Source: CAD feature listing. Evaluate the final solid. Frame: model axes, mm. A direction names the side the tool comes from. Give positions to 0.01 mm unless a question says otherwise; leave off trailing zeros. Loops run counter-clockwise (first coordinate to the right, second up) from the corner with the lowest first, then second, coordinate; pieces in that order, holes last. Notation, with made-up numbers: (47, -27.5) -> (56, -27.5) arc R18 ccw to (56, -3.5) -> close; hole circle Ø6 at (-22.5, 62). An arc over 180 degrees is marked (long way). Put each result on its own line as item: value.
```python
from build123d import *

# Parameters (mm, degrees)
SKETCH_1_W          = 74
SKETCH_1_H          = 42
SKETCH_1_R          = 1.275
EXTRUDE_1_DEPTH     = 2
SKETCH_2_R          = 1.525
CUT_EXTRUDE_1_DEPTH = 2
FILLET_1_R          = 2
SKETCH_3_W          = 30
SKETCH_3_H          = 22
EXTRUDE_2_DEPTH     = 2
SKETCH_4_R          = 2.025
CUT_EXTRUDE_2_DEPTH = 10
FILLET_2_R          = 2
CUT_EXTRUDE_3_DEPTH = 10
SKETCH_6_W          = 16
SKETCH_6_H          = 9
CUT_EXTRUDE_4_DEPTH = 10
FILLET_3_R          = 2


with BuildPart() as part:
    # 草图1 → 凸台-拉伸1 (new body)
    with BuildSketch(Plane.XY):
        Rectangle(SKETCH_1_W, SKETCH_1_H)
        with Locations((18, 18)):
            Circle(SKETCH_1_R, mode=Mode.SUBTRACT)
        with Locations((-18, 18)):
            Circle(SKETCH_1_R, mode=Mode.SUBTRACT)
        with Locations((-18, -18)):
            Circle(SKETCH_1_R, mode=Mode.SUBTRACT)
        with Locations((18, -18)):
            Circle(SKETCH_1_R, mode=Mode.SUBTRACT)
    extrude(amount=EXTRUDE_1_DEPTH)

    # 草图2 → 切除-拉伸1 (cut)
    with BuildSketch(Plane.XY.offset(2)):
        with Locations((34, 18)):
            Circle(SKETCH_2_R)
        with Locations((-34, 18)):
            Circle(SKETCH_2_R)
        with Locations((-34, -18)):
            Circle(SKETCH_2_R)
        with Locations((34, -18)):
            Circle(SKETCH_2_R)
    extrude(amount=-CUT_EXTRUDE_1_DEPTH, mode=Mode.SUBTRACT)

    # 圆角1
    fillet_1_edges = [part.edges().sort_by_distance(p)[0] for p in [
        (37, -21, 1),
        (-37, -21, 1),
        (-37, 21, 1),
        (37, 21, 1),
    ]]
    fillet(fillet_1_edges, radius=FILLET_1_R)

    # 草图3 → 凸台-拉伸2 (add)
    with BuildSketch(Plane.XY.offset(2)):
        with Locations((0, -21)):
            Rectangle(SKETCH_3_W, SKETCH_3_H)
    extrude(amount=-EXTRUDE_2_DEPTH)

    # 草图4 → 切除-拉伸2 (cut)
    with BuildSketch(Plane.XY.offset(2)):
        with Locations((12, -28)):
            Circle(SKETCH_4_R)
        with Locations((-12, -28)):
            Circle(SKETCH_4_R)
    extrude(amount=-CUT_EXTRUDE_2_DEPTH, mode=Mode.SUBTRACT)

    # 圆角2
    fillet_2_edges = [part.edges().sort_by_distance(p)[0] for p in [
        (15, -21, 1),
        (-15, -21, 1),
        (-15, -32, 1),
        (15, -32, 1),
    ]]
    fillet(fillet_2_edges, radius=FILLET_2_R)

    # 草图5 → 切除-拉伸3 (cut)
    with BuildSketch(Plane(origin=(0, 0, 0), x_dir=(-1, 0, 0), z_dir=(0, 0, -1))):
        Polygon((0, -2.18303115), (-27.010214515, -14), (27.010214515, -14), align=None)
        Polygon((-32, 11.81696885), (-32, -11.81696885), (-4.989785485, 0), align=None)
        Polygon((-27.010214515, 14), (0, 2.18303115), (27.010214515, 14), align=None)
        Polygon((32, 11.81696885), (4.989785485, 0), (32, -11.81696885), align=None)
    extrude(amount=-CUT_EXTRUDE_3_DEPTH, mode=Mode.SUBTRACT)

    # 草图6 → 切除-拉伸4 (cut)
    with BuildSketch(Plane(origin=(0, 0, 0), x_dir=(-1, 0, 0), z_dir=(0, 0, -1))):
        with Locations((0, -22.5)):
            Rectangle(SKETCH_6_W, SKETCH_6_H)
    extrude(amount=-CUT_EXTRUDE_4_DEPTH, mode=Mode.SUBTRACT)

    # 圆角3
    fillet_3_edges = [part.edges().sort_by_distance(p)[0] for p in [
        (0, 2.18303115, 1),
        (27.010214515, 14, 1),
        (-27.010214515, 14, 1),
        (32, -11.81696885, 1),
        (32, 11.81696885, 1),
        (4.989785485, 0, 1),
        (-4.989785485, 0, 1),
        (-32, 11.81696885, 1),
        (-32, -11.81696885, 1),
        (27.010214515, -14, 1),
        (0, -2.18303115, 1),
        (-27.010214515, -14, 1),
        (-8, -18, 1),
        (-8, -27, 1),
        (8, -27, 1),
        (8, -18, 1),
    ]]
    fillet(fillet_3_edges, radius=FILLET_3_R)


solid = part.part
```
(1) Draft query along Y for faces 3 (the flat face through (9.404, -6.297, 0.986)), 4 (the flat face through (-26, -21, 1)). Return one class per face: released by +Y, released by -Y, zero draft, split by the parting line, or undercut.
Calculated:
face 3: undercut
face 4: released by -Y
(2) Section B-B on x = -34. Return loops of the section in (y, z) (3 decimals), then the cut area to 3 significant figures.
Calculated:
outline: (-21, 0) -> (-19.525, 0) -> (-19.525, 2) -> (-21, 2) -> close; (-16.475, 0) -> (16.475, 0) -> (16.475, 2) -> (-16.475, 2) -> close; (19.525, 0) -> (21, 0) -> (21, 2) -> (19.525, 2) -> close
area: 71.8 mm²
(3) Section A-A on y = -28. Return loops of the section in (x, z) (3 decimals).
Calculated:
outline: (-15, 0) -> (-14.025, 0) -> (-14.025, 2) -> (-15, 2) -> close; (-9.975, 0) -> (9.975, 0) -> (9.975, 2) -> (-9.975, 2) -> close; (14.025, 0) -> (15, 0) -> (15, 2) -> (14.025, 2) -> close
(4) Reachability of faces 1 (the cylindrical face through (-31.07, -10.45, 1.01)), 2 (the cylindrical face through (36.4, -20.43, 1.01)) from +Z, -Z, +X, -X, +Y, -Y: full face, straight path, thin tool, end or side. Return the list, or none.
Calculated:
face 1: +Z, -Z
face 2: +Z, -Z, +X, -Y
(5) First-contact query: P1, Ø12, axis at x = -12, y = -16, coming from the -Z side; P2, Ø2, axis at x = -18, y = -18, coming from the +Z side; P3, Ø0.6, axis at x = -28.5, z = 1, coming from the -Y side; P4, Ø1, axis at y = -25, z = 1.5, coming from the +X side. Flat tips, straight axial feed; report the tip coordinate or a pass-through.
Calculated:
P1: stops at z = 0
P2: passes through
P3: stops at y = -21
P4: stops at x = 15
(6) Line query: probe 1 along Y at (x, z) = (34, 1.4) (3 decimals); probe 2 along X at (y, z) = (12, 0.45); probe 3 along Y at (x, z) = (-18, 0.65) (3 decimals). Output: solid intervals per line, ascending. Write a range as from..to.
Calculated:
probe 1: y = -21..-19.525, -16.475..16.475, 19.525..21
probe 2: x = -37..-19.45, 19.45..37
probe 3: y = -21..-19.275, -16.725..-13.923, -10.058..-5.692, 5.692..10.058, 13.923..16.725, 19.275..21
(7) Section D-D on z = 1.5. Give the number of separate pieces and of enclosed holes in the cut face, then the cut area to 3 significant figures.
Calculated:
separate pieces: 1
enclosed holes: 15
area: 2,010 mm²
(8) Section C-C on x = -26.5. Return loops of the section in (y, z).
Calculated:
outline: (-21, 0) -> (-9.41, 0) -> (-9.41, 2) -> (-21, 2) -> close; (9.41, 0) -> (21, 0) -> (21, 2) -> (9.41, 2) -> close
